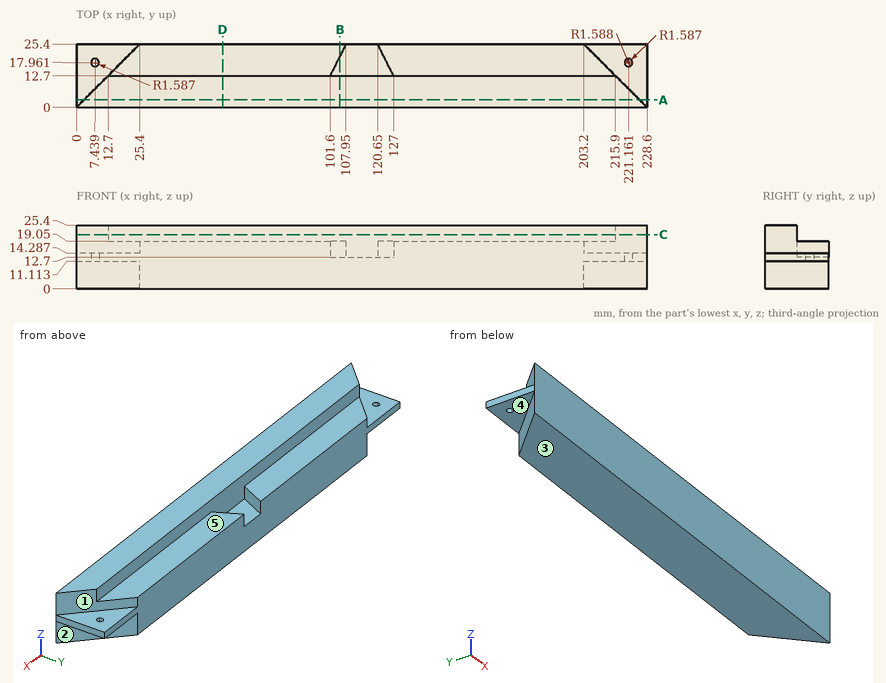
Print and shaded views of the part. All mm, measured from the part's lowest x, y and z. A direction names the side the tool comes from. Coordinates: 2 decimals unless noted, no trailing zeros. Write each loop counter-clockwise with the first axis right and the second up, starting at its lowest first coordinate (ties: lowest second). Pieces come first, ordered by that corner, then holes.
(1) 3-axis set-ups, long thin cutter, end or side, ignore diameter. For the marked faces 1, 2, 3, 4 and 5: which of +Z, -Z, +X, -X, +Y, -Y reach the whole face in a straight line?
(2) Flat gauge pins, fed straight in: pin 1 (2 mm diameter, centred on y = 12.5, z = 6.5, fed in from +X); pin 2 (1.5 mm diameter, centred on y = 21.5, z = 6, fed in from +X); pin 3 (12 mm diameter, centred on x = 56, y = 21, fed in from +Z). Where does each tip first touch, or does it go through?
(3) Cut at D-D, the plane x = 58.5. List the corners of the cut face in (y, z).
(4) Cut at B-B, the plane x = 105.5. List the corners of the cut face in (y, z), and give its area (3 significant figures).
(5) Cut at C-C, the plane z = 21.75. List the corners of the cut face in (x, y).
(6) Drill centre lines: probe 1 along Y at (x, z) = (120, 20); probe 2 along Z at (x, y) = (50, 18.25); probe 3 along X at (y, z) = (21.5, 17.5). Where is each one in solid material? Low to high.
(7) Cut at A-A, the plane y = 3. List the corners of the cut face in (x, z), and give its area (3 significant figures).
Geometry says:
1. face 1: +Z, +X, +Y
1. face 2: -Z, +X, +Y
1. face 3: -Z, +X, -X, +Y, -Y
1. face 4: -Z, -X, +Y
1. face 5: +Z, +X, -X, +Y
2. pin 1: stops at x = 217.1
2. pin 2: stops at x = 207.85
2. pin 3: stops at z = 19.05
3. outline: (0, 0) - (25.4, 0) - (25.4, 19.05) - (12.7, 19.05) - (12.7, 25.4) - (0, 25.4) - close
4. outline: (0, 0) - (25.4, 0) - (25.4, 19.05) - (20.5, 19.05) - (20.5, 12.7) - (12.7, 12.7) - (12.7, 25.4) - (0, 25.4) - close
4. area: 515 mm2
5. outline: (0, 0) - (228.6, 0) - (215.9, 12.7) - (12.7, 12.7) - close
6. probe 1: y = 0 to 12.7
6. probe 2: z = 0 to 19.05
6. probe 3: x = 21.5 to 106, 122.6 to 207.1
7. outline: (0, 11.11) - (3, 11.11) - (3, 0) - (225.6, 0) - (225.6, 11.11) - (228.6, 11.11) - (228.6, 14.29) - (225.6, 14.29) - (225.6, 25.4) - (3, 25.4) - (3, 14.29) - (0, 14.29) - close
7. area: 5,670 mm2
